Check sheet for the modelled part. Datum: model origin and axes. Units: mm. Face numbers are marked on the shaded views. Coordinates: 2 decimals unless noted, no trailing zeros. Write each loop counter-clockwise with the first axis right and the second up, starting at its lowest first coordinate (ties: lowest second). Pieces come first, ordered by that corner, then holes. Notation, with made-up numbers: (-12, 78.5) - (22, 78.5) arc R25 cw to (22, 111.5) - close; hole circle Ø3 at (-13, 16). An arc over 180 degrees is marked (long way). Write each question's results on one line, items separated by ' | '.
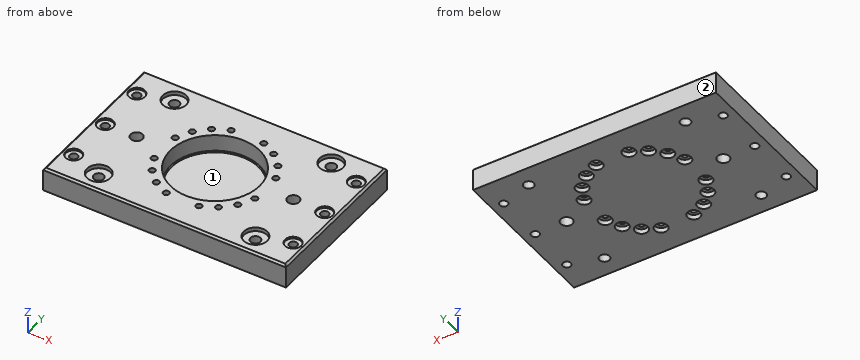
from build123d import *

# Parameters (mm, degrees)
SKETCH_1_W          = 124
SKETCH_1_H          = 80
EXTRUDE_1_DEPTH     = 12
SKETCH_2_R          = 22.75
CUT_EXTRUDE_1_DEPTH = 9
SKETCH_3_R          = 2.55
SKETCH_3_R_2        = 3.05
CUT_EXTRUDE_2_DEPTH = 75.752926364
SKETCH_4_R          = 2.05
CUT_EXTRUDE_3_DEPTH = 12
CHAMFER_1_SIZE      = 0.5
SKETCH_5_R          = 1.55
CUT_EXTRUDE_4_DEPTH = 12
SKETCH_6_R          = 3.25
CUT_EXTRUDE_5_DEPTH = 2.5
SKETCH_7_R          = 6
CUT_EXTRUDE_6_DEPTH = 2
SKETCH_8_R          = 4.1
CUT_EXTRUDE_7_DEPTH = 1
CHAMFER_2_SIZE      = 1


with BuildPart() as part:
    # Эскиз1 → Бобышка-Вытянуть1 (new body)
    with BuildSketch(Plane.XY):
        Rectangle(SKETCH_1_W, SKETCH_1_H)
    extrude(amount=EXTRUDE_1_DEPTH)

    # Эскиз2 → Вырез-Вытянуть1 (cut)
    with BuildSketch(Plane.XY.offset(12)):
        Circle(SKETCH_2_R)
    extrude(amount=-CUT_EXTRUDE_1_DEPTH, mode=Mode.SUBTRACT)

    # Эскиз3 → Вырез-Вытянуть2 (cut, through all)
    with BuildSketch(Plane.XY.offset(12)):
        with Locations((-40, 30)):
            Circle(SKETCH_3_R)
        with Locations((-40, 0)):
            Circle(SKETCH_3_R_2)
        with Locations((-40, -30)):
            Circle(SKETCH_3_R)
        with Locations((40, -30)):
            Circle(SKETCH_3_R)
        with Locations((40, 0)):
            Circle(SKETCH_3_R_2)
        with Locations((40, 30)):
            Circle(SKETCH_3_R)
    extrude(amount=-CUT_EXTRUDE_2_DEPTH, mode=Mode.SUBTRACT)

    # Эскиз4 → Вырез-Вытянуть3 (cut)
    with BuildSketch(Plane.XY.offset(12)):
        with Locations((-56, 25)):
            Circle(SKETCH_4_R)
        with Locations((-56, 0)):
            Circle(SKETCH_4_R)
        with Locations((-56, -25)):
            Circle(SKETCH_4_R)
        with Locations((56, -25)):
            Circle(SKETCH_4_R)
        with Locations((56, 0)):
            Circle(SKETCH_4_R)
        with Locations((56, 25)):
            Circle(SKETCH_4_R)
    extrude(amount=-CUT_EXTRUDE_3_DEPTH, mode=Mode.SUBTRACT)

    # Фаска1
    chamfer_1_edges = [part.edges().sort_by_distance(p)[0] for p in [
        (-22.75, 0, 3),
    ]]
    chamfer(chamfer_1_edges, length=CHAMFER_1_SIZE)

    # Эскиз5 → Вырез-Вытянуть4 (cut)
    with BuildSketch(Plane.XY.offset(12)):
        with Locations((-8.343458848, 25.67852594)):
            Circle(SKETCH_5_R)
        with Locations((8.343458848, 25.67852594)):
            Circle(SKETCH_5_R)
        with Locations((15.870201812, 21.843458848)):
            Circle(SKETCH_5_R)
        with Locations((21.843458848, 15.870201812)):
            Circle(SKETCH_5_R)
        with Locations((25.67852594, 8.343458848)):
            Circle(SKETCH_5_R)
        with Locations((25.67852594, -8.343458848)):
            Circle(SKETCH_5_R)
        with Locations((21.843458848, -15.870201812)):
            Circle(SKETCH_5_R)
        with Locations((15.870201812, -21.843458848)):
            Circle(SKETCH_5_R)
        with Locations((8.343458848, -25.67852594)):
            Circle(SKETCH_5_R)
        with Locations((-8.343458848, -25.67852594)):
            Circle(SKETCH_5_R)
        with Locations((-15.870201812, -21.843458848)):
            Circle(SKETCH_5_R)
        with Locations((-21.843458848, -15.870201812)):
            Circle(SKETCH_5_R)
        with Locations((-25.67852594, -8.343458848)):
            Circle(SKETCH_5_R)
        with Locations((-25.67852594, 8.343458848)):
            Circle(SKETCH_5_R)
        with Locations((-21.843458848, 15.870201812)):
            Circle(SKETCH_5_R)
        with Locations((-15.870201812, 21.843458848)):
            Circle(SKETCH_5_R)
    extrude(amount=-CUT_EXTRUDE_4_DEPTH, mode=Mode.SUBTRACT)

    # Эскиз6 → Вырез-Вытянуть5 (cut)
    with BuildSketch(Plane(origin=(0, 0, 0), x_dir=(-1, 0, 0), z_dir=(0, 0, -1))):
        with Locations((-8.343458848, 25.67852594)):
            Circle(SKETCH_6_R)
        with Locations((8.343458848, 25.67852594)):
            Circle(SKETCH_6_R)
        with Locations((15.870201812, 21.843458848)):
            Circle(SKETCH_6_R)
        with Locations((21.843458848, 15.870201812)):
            Circle(SKETCH_6_R)
        with Locations((25.67852594, 8.343458848)):
            Circle(SKETCH_6_R)
        with Locations((25.67852594, -8.343458848)):
            Circle(SKETCH_6_R)
        with Locations((21.843458848, -15.870201812)):
            Circle(SKETCH_6_R)
        with Locations((15.870201812, -21.843458848)):
            Circle(SKETCH_6_R)
        with Locations((8.343458848, -25.67852594)):
            Circle(SKETCH_6_R)
        with Locations((-8.343458848, -25.67852594)):
            Circle(SKETCH_6_R)
        with Locations((-15.870201812, -21.843458848)):
            Circle(SKETCH_6_R)
        with Locations((-21.843458848, -15.870201812)):
            Circle(SKETCH_6_R)
        with Locations((-25.67852594, -8.343458848)):
            Circle(SKETCH_6_R)
        with Locations((-25.67852594, 8.343458848)):
            Circle(SKETCH_6_R)
        with Locations((-21.843458848, 15.870201812)):
            Circle(SKETCH_6_R)
        with Locations((-15.870201812, 21.843458848)):
            Circle(SKETCH_6_R)
    extrude(amount=-CUT_EXTRUDE_5_DEPTH, mode=Mode.SUBTRACT)

    # Эскиз7 → Вырез-Вытянуть6 (cut)
    with BuildSketch(Plane.XY.offset(12)):
        with Locations((-40, -30)):
            Circle(SKETCH_7_R)
        with Locations((-40, 30)):
            Circle(SKETCH_7_R)
        with Locations((40, 30)):
            Circle(SKETCH_7_R)
        with Locations((40, -30)):
            Circle(SKETCH_7_R)
    extrude(amount=-CUT_EXTRUDE_6_DEPTH, mode=Mode.SUBTRACT)

    # Эскиз8 → Вырез-Вытянуть7 (cut)
    with BuildSketch(Plane.XY.offset(12)):
        with Locations((-56, 25)):
            Circle(SKETCH_8_R)
        with Locations((-56, 0)):
            Circle(SKETCH_8_R)
        with Locations((-56, -25)):
            Circle(SKETCH_8_R)
        with Locations((56, -25)):
            Circle(SKETCH_8_R)
        with Locations((56, 0)):
            Circle(SKETCH_8_R)
        with Locations((56, 25)):
            Circle(SKETCH_8_R)
    extrude(amount=-CUT_EXTRUDE_7_DEPTH, mode=Mode.SUBTRACT)

    # Фаска2
    chamfer_2_edges = [part.edges().sort_by_distance(p)[0] for p in [
        (-62, 0, 12),
        (0, -40, 12),
        (62, 0, 12),
        (0, 40, 12),
    ]]
    chamfer(chamfer_2_edges, length=CHAMFER_2_SIZE)


solid = part.part
1. Sectioned sample at A-A (x = -40). Record the cut outline in (y, z), then the cut area to 3 significant figures.
Values follow:
outline: (-40, 0) - (-32.55, 0) - (-32.55, 10) - (-36, 10) - (-36, 12) - (-39, 12) - (-40, 11) - close; (-27.45, 0) - (-3.05, 0) - (-3.05, 12) - (-24, 12) - (-24, 10) - (-27.45, 10) - close; (3.05, 0) - (27.45, 0) - (27.45, 10) - (24, 10) - (24, 12) - (3.05, 12) - close; (32.55, 0) - (40, 0) - (40, 11) - (39, 12) - (36, 12) - (36, 10) - (32.55, 10) - close | area: 736 mm^2
2. Material ranges on L1, parallel to Y at x = 40, z = 10.65; L2, parallel to Y at x = 41, z = 5; L3, parallel to Y at x = 18, z = 1, recorded low to high. Write a range as [from, to].
Values follow:
L1: y = [-40, -36], [-24, -3.05], [3.05, 24], [36, 40] | L2: y = [-40, -32.35], [-27.65, -2.88], [2.88, 27.65], [32.35, 40] | L3: y = [-40, -24.3], [-19.39, 19.39], [24.3, 40]
3. Sectioned sample at B-B (x = 0). Record the cut outline in (y, z).
Values follow:
outline: (-40, 0) - (40, 0) - (40, 11) - (39, 12) - (22.75, 12) - (22.75, 3.5) - (22.25, 3) - (-22.25, 3) - (-22.75, 3.5) - (-22.75, 12) - (-39, 12) - (-40, 11) - close
4. Draft check along X on the marked faces 1 and 2. Enter one of: pulls with the +X half, pulls with the -X half, needs draft (parallel to the pull), parting line crosses it, or undercut.
Values follow:
face 1: undercut | face 2: needs draft
5. Sectioned sample at C-C (y = 0). Give the number of separate pieces and of enclosed holes in the cut face, then the cut area to 3 significant figures.
Values follow:
separate pieces: 5 | enclosed holes: 0 | area: 825 mm^2
6. Go/stop test with flat-tipped pins: pin 1 (5 mm diameter, centred on x = -8.34, y = 25.68, fed in from -Z); pin 2 (2.5 mm diameter, centred on x = 57.5, y = -1.5, fed in from +Z); pin 3 (22 mm diameter, centred on x = 3, y = 6.5, fed in from +Z). Record where each tip stops, or that it passes through.
Values follow:
pin 1: stops at z = 2.5 | pin 2: stops at z = 11 | pin 3: stops at z = 3
